Design review of the part shown in the three views and the two pictorial views. Dimensions are in mm from the part's minimum x, y and z. A direction names the side the tool comes from. Give positions to 0.01 mm unless a question says otherwise; leave off trailing zeros. Loops run counter-clockwise (first coordinate to the right, second up) from the corner with the lowest first, then second, coordinate; pieces in that order, holes last. Notation, with made-up numbers: (-18, 79) - (-8, 79) arc R23 cw to (-8, 117) - close; hole circle Ø11 at (28, -40). An arc over 180 degrees is marked (long way). Answer as a JSON object with one key per item and string values.
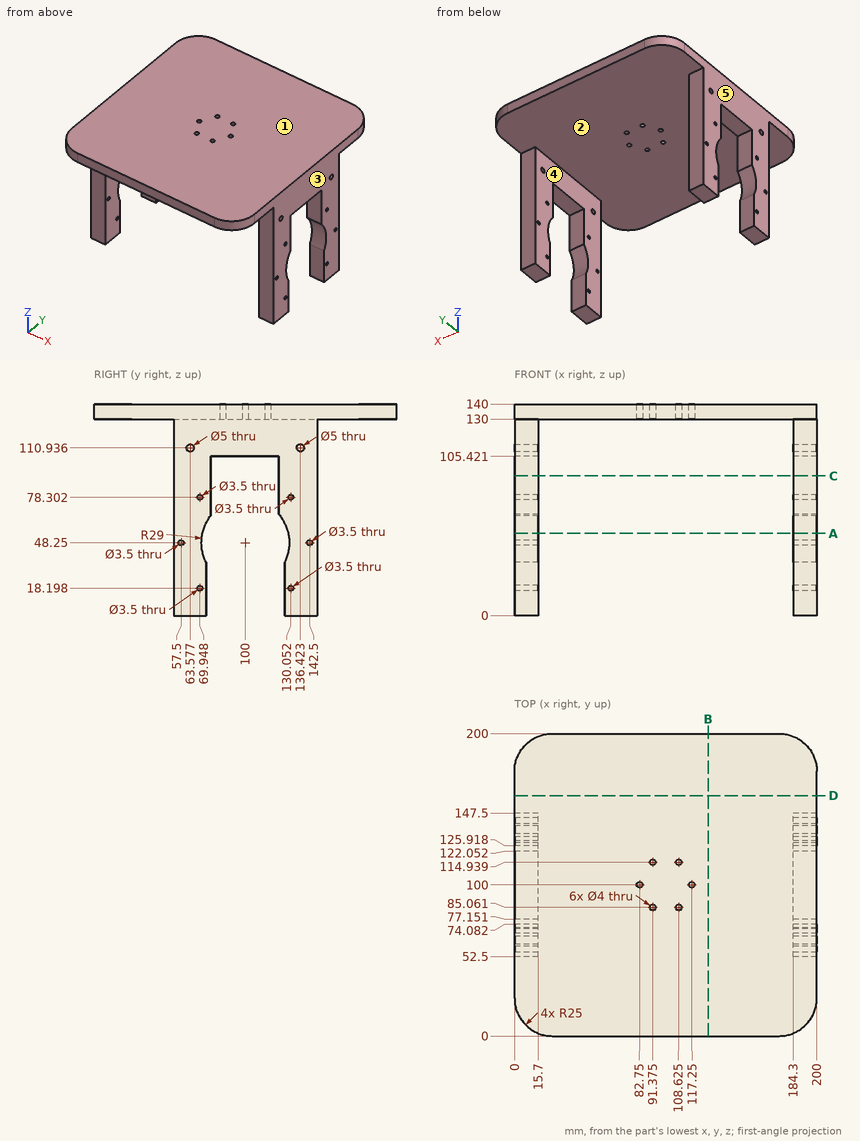
Q1. The part is to be moulded in two halves that separate along X. For the marked faces 1, 2 and 3, say which applies: +X half, -X half, draft (parallel to the pull), parting line (faces both ways), or undercut.
Results:
{"face 1": "draft", "face 2": "undercut", "face 3": "+X half"}
Q2. To check wall thickness, follow probe 1 along Z at (x, y) = (9, 142.5); probe 2 along Y at (x, z) = (117.25, 134.5); probe 3 along Z at (x, y) = (173, 98.5). State the ranges of each line that lie inside material, in increasing order. Write a range as [from, to].
Results:
{"probe 1": "z = [0, 46.5], [50, 140]", "probe 2": "y = [0, 98], [102, 200]", "probe 3": "z = [130, 140]"}
Q3. Consider section A-A, the plane z = 54.5. State the section outline as (x, y) points, plus the area to 3 significant figures.
Results:
{"outline": "(0, 52.5) - (15.7, 52.5) - (15.7, 71.68) - (0, 71.68) - close; (0, 128.32) - (15.7, 128.32) - (15.7, 147.5) - (0, 147.5) - close; (184.3, 52.5) - (200, 52.5) - (200, 71.68) - (184.3, 71.68) - close; (184.3, 128.32) - (200, 128.32) - (200, 147.5) - (184.3, 147.5) - close", "area": "1,200 mm^2"}
Q4. Consider section B-B, the plane x = 128. State the section outline as (y, z) points.
Results:
{"outline": "(0, 130) - (200, 130) - (200, 140) - (0, 140) - close"}
Q5. Clearance check with flat-ended pins moving along their axes: pin 1 Ø8 at (x, z) = (191.5, 93) entering from -Y; pin 2 Ø12.5 at (x, y) = (193, 101) entering from -Z; pin 3 Ø4.5 at (x, z) = (188.5, 88) entering from +Y. State where each tip first meets the part, or that it passes through.
Results:
{"pin 1": "stops at y = 52.5", "pin 2": "stops at z = 105.42", "pin 3": "stops at y = 147.5"}
Q6. For the marked faces 4 and 5, list the 3-axis set-ups (+Z, -Z, +X, -X, +Y, -Y) from which the entire face can be reached by the end or side of a thin tool; tool diameter is ignored.
Results:
{"face 4": "-Z, +Y, -Y", "face 5": "+Z, -Z, -X, +Y, -Y"}
Q7. Consider section C-C, the plane z = 92.5. State the section outline as (x, y) points.
Results:
{"outline": "(0, 52.5) - (15.7, 52.5) - (15.7, 77.15) - (0, 77.15) - close; (0, 122.05) - (15.7, 122.05) - (15.7, 147.5) - (0, 147.5) - close; (184.3, 52.5) - (200, 52.5) - (200, 77.15) - (184.3, 77.15) - close; (184.3, 122.05) - (200, 122.05) - (200, 147.5) - (184.3, 147.5) - close"}
